```python
from build123d import *

# Parameters (mm, degrees)
AXLE_BASE_SKETCH_R        = 26
AXLE_DEPTH                = 77.5
GUARD_BASE_R              = 37.5
GUARD_DEPTH               = 5
INNER_AXLE_HOLE_BASE_R    = 8.5
INNER_AXLE_HOLE_DEPTH     = 83.5
BEND_START                = -65.25
BEND_ROOM_BASE_W          = 1.5
BEND_ROOM_BASE_H          = 75
BEND_ROOM_1_DEPTH         = 65.25
BEND_ROOM_2_COUNT         = 2
BEND_ROOM_2_ANGLE         = 90
EASY_REMOVAL_CHAMFER_SIZE = 4


with BuildPart() as part:
    # Axle base sketch → Axle (new body)
    with BuildSketch(Plane.XY):
        Circle(AXLE_BASE_SKETCH_R)
    extrude(amount=AXLE_DEPTH)

    # Guard base → Guard (add)
    with BuildSketch(Plane(origin=(0, 0, 0), x_dir=(-1, 0, 0), z_dir=(0, 0, -1))):
        Circle(GUARD_BASE_R)
    extrude(amount=GUARD_DEPTH)

    # Inner axle hole base → Inner axle hole (cut, through all)
    with BuildSketch(Plane.XY.offset(77.5)):
        Circle(INNER_AXLE_HOLE_BASE_R)
    extrude(amount=-INNER_AXLE_HOLE_DEPTH, mode=Mode.SUBTRACT)

    # Mate ring base → Mate rings (revolve)
    with BuildSketch(Plane(origin=(0, 0, 0), x_dir=(1, 0, 0), z_dir=(0, 1, 0))):
        Polygon((26, -77.5), (26.75, -76.75), (26.75, -76), (26, -75.25), align=None)
        Polygon((26, -71.75), (26.75, -71), (26.75, -70.25), (26, -69.5), align=None)
    revolve(axis=Axis((0, 0, 0), (0, 0, -1)))

    # Inner mass remove base → Inner mass remove (revolve, cut)
    with BuildSketch(Plane(origin=(0, 0, 0), x_dir=(0, 0, -1), z_dir=(1, 0, 0))):
        Polygon((-77.5, 0), (-60.25, -17.25), (-12.25, -17.25), (5, 0), align=None)
    revolve(axis=Axis((0, 0, 0), (0, 0, -1)), mode=Mode.SUBTRACT)

    # Bend room base → Bend room 1 (cut)
    with BuildSketch(Plane.XY.offset(77.5).offset(BEND_START)):
        Rectangle(BEND_ROOM_BASE_W, BEND_ROOM_BASE_H)
    bend_room_1 = extrude(amount=BEND_ROOM_1_DEPTH, mode=Mode.SUBTRACT)

    # Bend room 2: Bend room 1 ×2 about axis
    bend_room_2_axis = Axis((0, 0, 0), (0, 0, -1))
    for i in range(1, BEND_ROOM_2_COUNT):
        add(bend_room_1.rotate(bend_room_2_axis, i * BEND_ROOM_2_ANGLE / (BEND_ROOM_2_COUNT - 1)), mode=Mode.SUBTRACT)

    # Easy removal chamfer
    easy_removal_chamfer_edges = [part.edges().sort_by_distance(p)[0] for p in [
        (37.5, 0, 0),
    ]]
    chamfer(easy_removal_chamfer_edges, length=EASY_REMOVAL_CHAMFER_SIZE)


solid = part.part
```
Geometry: final body of the model. Coordinates: model frame, mm. A direction names the side the tool comes from. Round coordinates to 2 decimals unless told otherwise and drop trailing zeros. Order: outer loops, then holes, each group sorted by start corner. A loop starts at its lowest first (then second) coordinate and runs counter-clockwise, first axis right, second up. Notation, with made-up numbers: (-20.5, 4) -> (7.5, 4) arc R17 cw to (7.5, 16) -> close; hole circle Ø2 at (72, -18.5). An arc over 180 degrees is marked (long way). Use one line per item in the form item = value. Start each with the question number.
1. Cut plane B-B (z = 10). Return the cut outline in (x, y), then the cut area to 3 significant figures.
2. Line query: probe 1 along Y at (x, z) = (1, 31.5); probe 2 along X at (y, z) = (-18, 43); probe 3 along X at (y, z) = (-7, 65). Output: solid intervals per line, ascending.
3. Pin query (flat end, axial travel): pin 1 Ø1.2 at (x, y) = (-23.5, 0) entering from +Z; pin 2 Ø5.5 at (x, z) = (18, 50.5) entering from +Y; pin 3 Ø5 at (x, z) = (-16.5, 9.5) entering from +Y; pin 4 Ø0.8 at (x, y) = (-0.5, -20) entering from +Z. Return the tip coordinate at first contact, or that it passes through.
4. Draft query along Y for faces 1 (the face through (-12.324, 12.07, 35.914)), 2 (the face through (-18.58, -18.19, 73.48)), 3 (the face through (-14, -13, 77.5)). Return one class per face: pulls with the +Y half, pulls with the -Y half, needs draft (parallel to the pull), parting line crosses it, or undercut.
5. Cut plane A-A (z = 54). Return the cut outline in (x, y).
6. Reachability of faces 4 (the face through (-18.19, 18.58, 73.48)), 5 (the face through (18.273, 18.664, 69.62)), 6 (the face through (12.07, 12.324, 35.914)), 7 (the face through (18.713, 19.115, 76.37)), 8 (the face through (-18.713, -19.115, 70.62)) from +Z, -Z, +X, -X, +Y, -Y: full face, straight path, thin tool, end or side. Return the list, or none.
Solution:
q1.outline = circle Ø52 at (0, 0); hole circle Ø30 at (0, 0)
q1.area = 1,420 mm^2
q2.probe_1 = -25.98 to -17.22, 17.22 to 25.98
q2.probe_2 = -18.76 to -0.75, 0.75 to 18.76
q2.probe_3 = -25.04 to -10.36, 10.36 to 25.04
q3.pin_1 = 12.25
q3.pin_2 = 21.06
q3.pin_3 = 21.91
q3.pin_4 = 77.5
q4.face_1 = undercut
q4.face_2 = pulls with the -Y half
q4.face_3 = needs draft
q5.outline = (-25.99, -0.75) arc R26 ccw to (-0.75, -25.99) -> (-0.75, -17.23) arc R17.25 cw to (-17.23, -0.75) -> close; (-25.99, 0.75) -> (-17.23, 0.75) arc R17.25 cw to (-0.75, 17.23) -> (-0.75, 25.99) arc R26 ccw to start; (0.75, -25.99) arc R26 ccw to (25.99, -0.75) -> (17.23, -0.75) arc R17.25 cw to (0.75, -17.23) -> close; (0.75, 17.23) arc R17.25 cw to (17.23, 0.75) -> (25.99, 0.75) arc R26 ccw to (0.75, 25.99) -> close
q6.face_4 = -X, +Y
q6.face_5 = +X, +Y
q6.face_6 = none
q6.face_7 = +Z, +X, +Y
q6.face_8 = +Z, -X, -Y
